The model under review builds one solid part; all positions refer to its coordinate system, in mm. Face numbers are marked on the shaded views. A direction names the side the tool comes from. Coordinates: 2 decimals unless noted, no trailing zeros. Order: outer loops, then holes, each group sorted by start corner. A loop starts at its lowest first (then second) coordinate and runs counter-clockwise, first axis right, second up. Notation, with made-up numbers: (63, 9) -> (121, 9) arc R23 ccw to (121, 28) -> close; hole circle Ø10 at (55.5, -31). An arc over 180 degrees is marked (long way). Use one line per item in the form item = value. Start each with the question number.
(1) For the marked faces 4 and 5, list the 3-axis set-ups (+Z, -Z, +X, -X, +Y, -Y) from which the entire face can be reached by the end or side of a thin tool; tool diameter is ignored.
(2) Take a section at B-B (y = -5.5). State the section outline as (x, z) points, then the cut area to 3 significant figures.
(3) Take a section at A-A (z = -18). State the section outline as (x, y) points.
(4) Mouldability with a two-part tool opening along Z and no side actions: class the marked faces 1, 2 and 3 as +Z half, -Z half, draft (parallel to the pull), parting line (faces both ways), or undercut.
(5) Wall thickness on line 1 along X through (y, z) = (-3.75, -14); line 2 along X through (y, z) = (-6.25, -21): over which ranges is each line inside the solid? List them lowest first.
```python
from build123d import *

# Parameters (mm, degrees)
SKETCH1_W           = 100
SKETCH1_H           = 50
BOSS_EXTRUDE1_DEPTH = 25
CUT_EXTRUDE1_DEPTH  = 10


with BuildPart() as part:
    # Sketch1 → Boss-Extrude1 (new body)
    with BuildSketch(Plane(origin=(0, 0, 0), x_dir=(1, 0, 0), z_dir=(0, 1, 0))):
        Rectangle(SKETCH1_W, SKETCH1_H)
    extrude(amount=-BOSS_EXTRUDE1_DEPTH)

    # Sketch2 → Cut-Extrude1 (cut)
    with BuildSketch(Plane(origin=(0, 0, 0), x_dir=(1, 0, 0), z_dir=(0, 1, 0))):
        with BuildLine():
            Line((33.7, 20.878679656), (33.7, 10.821320344))
            ThreePointArc((33.7, 10.821320344), (33.7, 8.7), (35.821320344, 8.7))
            Line((35.821320344, 8.7), (45.878679656, 8.7))
            ThreePointArc((45.878679656, 8.7), (48, 8.7), (48, 10.821320344))
            Line((48, 10.821320344), (48, 20.878679656))
            ThreePointArc((48, 20.878679656), (48, 23), (45.878679656, 23))
            Line((45.878679656, 23), (35.821320344, 23))
            ThreePointArc((35.821320344, 23), (33.7, 23), (33.7, 20.878679656))
        make_face()
    extrude(amount=-CUT_EXTRUDE1_DEPTH, mode=Mode.SUBTRACT)


solid = part.part
```
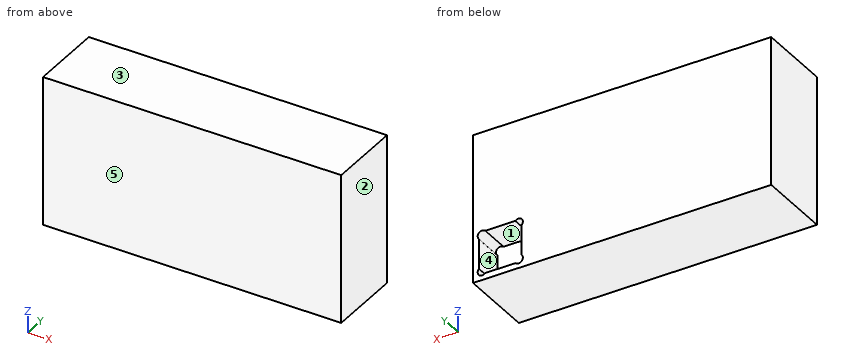
Findings:
q1.face_4 = +Y
q1.face_5 = +Z, -Z, +X, -X, -Y
q2.outline = (-50, -25) -> (50, -25) -> (50, 25) -> (-50, 25) -> close; hole (33.7, -20.88) arc R1.5 ccw to (35.82, -23) -> (45.88, -23) arc R1.5 ccw to (48, -20.88) -> (48, -10.82) arc R1.5 ccw to (45.88, -8.7) -> (35.82, -8.7) arc R1.5 ccw to (33.7, -10.82) -> close
q2.area = 4,790 mm²
q3.outline = (-50, -25) -> (50, -25) -> (50, 0) -> (48, 0) -> (48, -10) -> (33.7, -10) -> (33.7, 0) -> (-50, 0) -> close
q4.face_1 = undercut
q4.face_2 = draft
q4.face_3 = +Z half
q5.line_1 = -50 to 33.7, 48 to 50
q5.line_2 = -50 to 33.59, 48.11 to 50
